from build123d import *

# Parameters (mm, degrees)
F0_R     = 4.6
F1_DEPTH = 3


with BuildPart() as f1:
    # F0 (on Top) → F1 (new body)
    with BuildSketch(Plane.XY):
        with BuildLine():
            ThreePointArc((-11, 0), (0, -11), (11, 0))
            ThreePointArc((11, 0), (0, 11), (-11, 0))
        make_face()
        with Locations((-22, 0)):
            Circle(F0_R)
        with BuildLine():
            ThreePointArc((-14.432727, 4.086121), (-30.6, 0), (-14.432727, -4.086121))
            ThreePointArc((-14.432727, -4.086121), (-7.5, -12.990381), (3.677679, -14.542169))
            ThreePointArc((3.677679, -14.542169), (15.3, -26.500377), (10.755048, -10.456048))
            ThreePointArc((10.755048, -10.456048), (15, 0), (10.755048, 10.456048))
            ThreePointArc((10.755048, 10.456048), (15.3, 26.500377), (3.677679, 14.542169))
            ThreePointArc((3.677679, 14.542169), (-7.5, 12.990381), (-14.432727, 4.086121))
        make_face()
        with Locations((11, -19.052559)):
            Circle(F0_R, mode=Mode.SUBTRACT)
        with Locations((-22, 0)):
            Circle(F0_R, mode=Mode.SUBTRACT)
        with BuildLine():
            ThreePointArc((-11, 0), (0, 11), (11, 0))
            ThreePointArc((11, 0), (0, -11), (-11, 0))
        make_face(mode=Mode.SUBTRACT)
        with Locations((11, 19.052559)):
            Circle(F0_R, mode=Mode.SUBTRACT)
    extrude(amount=F1_DEPTH)


solid = f1.part
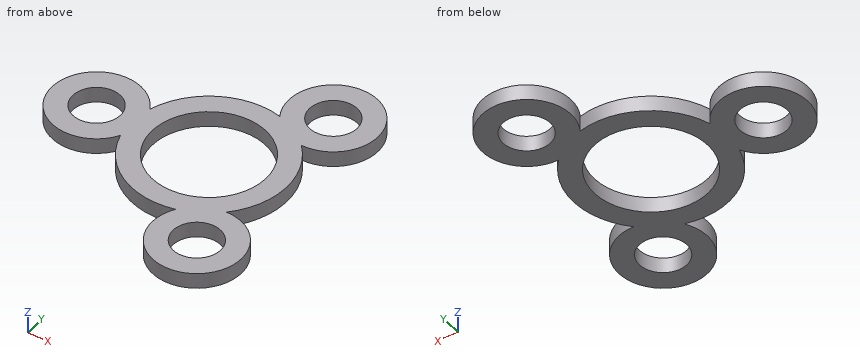
Design review of the part built by this model. Coordinates are the model's own, in mm. Give positions to 0.01 mm unless a question says otherwise; leave off trailing zeros. Loops run counter-clockwise (first coordinate to the right, second up) from the corner with the lowest first, then second, coordinate; pieces in that order, holes last. Notation, with made-up numbers: (66.5, -35.75) -> (95.5, -35.75) arc R22 ccw to (95.5, -16.75) -> close; hole circle Ø4 at (12.25, 1). An arc over 180 degrees is marked (long way). One line per question, with ' | ' between items. Start each with the question number.
(1) We need section B-B (x = -22). State the section outline as (y, z) points.
(2) We need section C-C (y = -22). State the section outline as (x, z) points.
(3) Insertion check: P1, Ø10.5, axis at x = 11, y = 19.05, coming from the +Z side; P2, Ø5.5, axis at x = -22, y = 0, coming from the -Z side; P3, Ø1.5, axis at x = -22, z = 1, coming from the +Y side. Each pin has a flat end and moves straight along its axis. Give the tip position at first contact, or say it passes through.
(4) We need section A-A (y = 0). State the section outline as (x, z) points.
(5) For line 1 (Y direction, x = -22, z = 1.2); line 2 (Y direction, x = 8, z = 1.3); line 3 (X direction, y = 19, z = 2.1), list the stretches that pass through material, from the lowest coordinate up.
(6) We need section D-D (x = 7). State the section outline as (y, z) points.
The answers:
1) outline: (-8.6, 0) -> (-4.6, 0) -> (-4.6, 3) -> (-8.6, 3) -> close; (4.6, 0) -> (8.6, 0) -> (8.6, 3) -> (4.6, 3) -> close
2) outline: (2.92, 0) -> (7.47, 0) -> (7.47, 3) -> (2.92, 3) -> close; (14.53, 0) -> (19.08, 0) -> (19.08, 3) -> (14.53, 3) -> close
3) P1: stops at z = 3 | P2: passes through | P3: stops at y = 8.6
4) outline: (-30.6, 0) -> (-26.6, 0) -> (-26.6, 3) -> (-30.6, 3) -> close; (-17.4, 0) -> (-11, 0) -> (-11, 3) -> (-17.4, 3) -> close; (11, 0) -> (15, 0) -> (15, 3) -> (11, 3) -> close
5) line 1: y = -8.6 to -4.6, 4.6 to 8.6 | line 2: y = -27.11 to -22.54, -15.57 to -7.55, 7.55 to 15.57, 22.54 to 27.11 | line 3: x = 2.4 to 6.4, 15.6 to 19.6
6) outline: (-26.67, 0) -> (-21.32, 0) -> (-21.32, 3) -> (-26.67, 3) -> close; (-16.78, 0) -> (-8.49, 0) -> (-8.49, 3) -> (-16.78, 3) -> close; (8.49, 0) -> (16.78, 0) -> (16.78, 3) -> (8.49, 3) -> close; (21.32, 0) -> (26.67, 0) -> (26.67, 3) -> (21.32, 3) -> close
